Input: part model. Units: mm. Frame: model coordinates. A direction names the side the tool comes from. Coordinates: 2 decimals unless noted, no trailing zeros. Order: outer loops, then holes, each group sorted by start corner. A loop starts at its lowest first (then second) coordinate and runs counter-clockwise, first axis right, second up. Notation, with made-up numbers: (46.5, -18.75) - (81.5, -18.75) arc R20 ccw to (81.5, -12.75) - close; hole circle Ø9 at (8, -0.5). An arc over 180 degrees is marked (long way). Answer as CSV lines item,"result". Start each with the question number.
Item 1: Section B-B (x = 7.5). Output: boundary loops of the cut face in (y, z).
Item 2: Section A-A (y = -37.5). Output: boundary loops of the cut face in (x, z), and give its area (3 significant figures).
Item 3: Section D-D (y = 0). Output: boundary loops of the cut face in (x, z).
Item 4: First-contact query: pin 1 (7.5 mm diameter, centred on y = -37.5, z = 0, fed in from -X); pin 2 (4 mm diameter, centred on x = 10.5, y = 26, fed in from +Z); pin 3 (10.5 mm diameter, centred on y = 0, z = -37.5, fed in from +X). Flat tips, straight axial feed; report the tip coordinate or a pass-through.
Item 5: Access query for faces 1 (the cylindrical face through (6.958, 49.592, -11.012)), 2 (the flat face through (21, -42, -27.5)), 3 (the cylindrical face through (12.381, 34.498, -1.245)). Directions: +Z, -Z, +X, -X, +Y, -Y. A direction counts if a zero-diameter tool reaches every point of the face in a straight line with its end or side. Return the directions, or none.
Item 6: Draft query along Z for faces 4 (the conical face through (21.2, 34.2, 1)), 5 (the flat face through (0, 0, 0)), 6 (the cylindrical face through (15.42, -2.75, -62.44)), 7 (the cylindrical face through (15.58, -59.2, 14.97)). Return one class per face: +Z half, -Z half, draft (parallel to the pull), parting line (faces both ways), or undercut.
Item 7: Material intervals for line 1 along Z through (x, y) = (8.25, 0); line 2 along Z through (x, y) = (15.75, 0); line 3 along Y through (x, z) = (18.25, 38), sorted ascending.
from build123d import *

# Parameters (mm, degrees)
F2_R     = 4
F3_DEPTH = 25
F4_R     = 3.25
F5_DEPTH = 25
F6_SIZE  = 3


# Not quite as in the source:
# - a feature names something its author has since deleted; it is built from what else it names


with BuildPart() as f1:
    # F0 (on Front) → F1 (revolve)
    with BuildSketch(Plane.XZ):
        Polygon((0, 9.55), (0, 0), (17.623, 0), (24, 0), (24, 50), (21, 50), (21, 62.5), (10, 62.5), (10, 50.8), (4, 50.8), (4, 9.55), align=None)
    revolve(axis=Axis((8.8115, 0, 0), (1, 0, 0)))

    # F2 (on face) → F3 (cut)
    with BuildSketch(Plane.YZ.offset(21)):
        with BuildLine():
            ThreePointArc((44.4111525448, 40.4111525448), (38.8804188154, 44.1066706749), (37.5827254201, 37.5827254201))
            ThreePointArc((37.5827254201, 37.5827254201), (41.9418862743, 36.7156344148), (44.4111525448, 40.4111525448))
        make_face()
        with Locations((-55.2026609724, 14.7915084276)):
            Circle(F2_R)
        with Locations((14.7915084276, -55.2026609724)):
            Circle(F2_R)
    extrude(amount=-F3_DEPTH, mode=Mode.SUBTRACT)

    # F4 (on face) → F5 (cut)
    with BuildSketch(Plane(origin=(4, 0, 0), x_dir=(0, -1, 0), z_dir=(-1, 0, 0))):
        with Locations((0, 37.5)):
            Circle(F4_R)
        with Locations((-37.5, 0)):
            Circle(F4_R)
        with Locations((0, -37.5)):
            Circle(F4_R)
        with Locations((37.5, 0)):
            Circle(F4_R)
    extrude(amount=-F5_DEPTH, mode=Mode.SUBTRACT)

    # F6
    f6_edges = [f1.edges().sort_by_distance(p)[0] for p in [
        (24, -34.25, 0),
        (24, 3.25, 37.5),
        (24, 40.75, 0),
        (24, 3.25, -37.5),
    ]]
    chamfer(f6_edges, length=F6_SIZE)


solid = f1.part
Determined:
1,outline,"circle Ø101.6 at (0, 0); hole circle Ø6.5 at (-37.5, 0); hole circle Ø6.5 at (0, -37.5); hole circle Ø6.5 at (0, 37.5); hole circle Ø6.5 at (37.5, 0)"
2,outline,"(4, -34.27) - (10, -34.27) - (10, -50) - (21, -50) - (21, -33.07) - (24, -33.07) - (24, -6.25) - (21, -3.25) - (4, -3.25) - close; (4, 3.25) - (21, 3.25) - (24, 6.25) - (24, 33.07) - (21, 33.07) - (21, 50) - (10, 50) - (10, 34.27) - (4, 34.27) - close"
2,area,"1,570 mm^2"
3,outline,"(0, -9.55) - (4, -9.55) - (4, -34.25) - (21, -34.25) - (24, -31.25) - (24, 31.25) - (21, 34.25) - (4, 34.25) - (4, 9.55) - (0, 9.55) - close; (4, -50.8) - (10, -50.8) - (10, -62.5) - (21, -62.5) - (21, -50) - (24, -50) - (24, -43.75) - (21, -40.75) - (4, -40.75) - close; (4, 40.75) - (21, 40.75) - (24, 43.75) - (24, 50) - (21, 50) - (21, 62.5) - (10, 62.5) - (10, 50.8) - (4, 50.8) - close"
4,pin 1,"stops at x = 4"
4,pin 2,"stops at z = 57.71"
4,pin 3,"stops at x = 23"
5,face 1,"-X"
5,face 2,"+X"
5,face 3,"+X, -X"
6,face 4,"undercut"
6,face 5,"draft"
6,face 6,"parting line"
6,face 7,"undercut"
7,line 1,"z = -50.8 to -40.75, -34.25 to 34.25, 40.75 to 50.8"
7,line 2,"z = -62.5 to -40.75, -34.25 to 34.25, 40.75 to 62.5"
7,line 3,"y = -49.62 to -3.21, 3.21 to 37.22, 43.6 to 49.62"
